Source: CAD feature listing. Evaluate the final solid. Frame: model axes, mm. Face numbers are marked on the shaded views. A direction names the side the tool comes from. Round coordinates to 2 decimals unless told otherwise and drop trailing zeros. Order: outer loops, then holes, each group sorted by start corner. A loop starts at its lowest first (then second) coordinate and runs counter-clockwise, first axis right, second up.
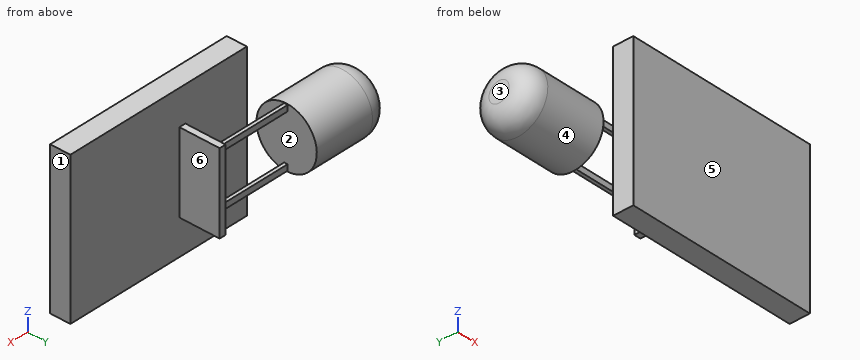
```python
from build123d import *

# Parameters (mm, degrees)
ESQUISSE1_W        = 19
ESQUISSE1_H        = 15
BOSS_EXTRU_1_DEPTH = 2
ESQUISSE2_W        = 0.642500129
ESQUISSE2_H        = 8.011173479
BOSS_EXTRU_2_DEPTH = 4
ESQUISSE3_W        = 0.58049635
ESQUISSE3_H        = 0.338622871
BOSS_EXTRU_3_DEPTH = 8
ESQUISSE4_R        = 3
BOSS_EXTRU_4_DEPTH = 8
CONG_1_R           = 2


with BuildPart() as part:
    # Esquisse1 → Boss.-Extru.1 (new body)
    with BuildSketch(Plane(origin=(0, 0, 0), x_dir=(1, 0, 0), z_dir=(0, 1, 0))):
        Rectangle(ESQUISSE1_W, ESQUISSE1_H)
    extrude(amount=BOSS_EXTRU_1_DEPTH)

    # Esquisse2 → Boss.-Extru.2 (add)
    with BuildSketch(Plane(origin=(0, 2, 0), x_dir=(1, 0, 0), z_dir=(0, 1, 0))):
        with Locations((-2.562175711, -0.012775057)):
            Rectangle(ESQUISSE2_W, ESQUISSE2_H)
    extrude(amount=BOSS_EXTRU_2_DEPTH)

    # Esquisse3 → Boss.-Extru.3 (add)
    with BuildSketch(Plane.ZY.offset(2.883425775)):
        with Locations((-2.628358474, 4.603596233)):
            Rectangle(ESQUISSE3_W, ESQUISSE3_H)
    boss_extru_3 = extrude(amount=BOSS_EXTRU_3_DEPTH)

    # Symétrie1: Boss.-Extru.3 across plane
    add(boss_extru_3.mirror(Plane.XY))

    # Esquisse4 → Boss.-Extru.4 (add)
    with BuildSketch(Plane.ZY.offset(10.883425775)):
        with Locations((0, 4.67632737)):
            Circle(ESQUISSE4_R)
    extrude(amount=BOSS_EXTRU_4_DEPTH)

    # Congé1
    cong_1_edges = [part.edges().sort_by_distance(p)[0] for p in [
        (-18.883425775, 4.67632737, -3),
    ]]
    fillet(cong_1_edges, radius=CONG_1_R)


solid = part.part
```
1. Section A-A on x = -5. Return loops of the section in (y, z).
2. First-contact query: pin 1 (3 mm diameter, centred on x = -7.5, z = -5, fed in from +Y); pin 2 (1.2 mm diameter, centred on y = 5, z = 1, fed in from +X); pin 3 (1.5 mm diameter, centred on x = -4.5, z = -3, fed in from +Y). Flat tips, straight axial feed; report the tip coordinate or a pass-through.
3. Section C-C on x = 6.75. Return loops of the section in (y, z).
4. Access query for the marked faces 5 and 6. Directions: +Z, -Z, +X, -X, +Y, -Y. A direction counts if a zero-diameter tool reaches every point of the face in a straight line with its end or side. Return the directions, or none.
5. Pull-direction query (X, two-part tool) for the marked faces 1, 2, 3 and 4; classes: released by +X, released by -X, zero draft, split by the parting line, or undercut.
6. Line query: line 1 along Z through (x, y) = (-7.75, 4.5); line 2 along Y through (x, z) = (8, -5); line 3 along X through (y, z) = (0.75, -3). Output: solid intervals per line, ascending.
7. Section B-B on z = 5.75. Return loops of the section in (x, y).
Result:
1. outline: (0, -7.5) - (2, -7.5) - (2, 7.5) - (0, 7.5) - close; (4.43, -2.92) - (4.77, -2.92) - (4.77, -2.34) - (4.43, -2.34) - close; (4.43, 2.34) - (4.77, 2.34) - (4.77, 2.92) - (4.43, 2.92) - close
2. pin 1: stops at y = 2
2. pin 2: stops at x = -2.24
2. pin 3: stops at y = 4.77
3. outline: (0, -7.5) - (2, -7.5) - (2, 7.5) - (0, 7.5) - close
4. face 5: +Z, -Z, +X, -X, -Y
4. face 6: +Z, -Z, +X, +Y
5. face 1: released by +X
5. face 2: undercut
5. face 3: released by -X
5. face 4: zero draft
6. line 1: z = -2.92 to -2.34, 2.34 to 2.92
6. line 2: y = 0 to 2
6. line 3: x = -9.5 to 9.5
7. outline: (-9.5, 0) - (9.5, 0) - (9.5, 2) - (-9.5, 2) - close
